```python
from build123d import *

# Parameters (mm, degrees)
F0_R          = 9
F1_DEPTH      = 25
F2_R          = 5
F3_DEPTH      = 10
F4_R          = 4
F5_DEPTH      = 8
F6_R          = 2
F7_DEPTH      = 9.001
F7_DEPTH_BACK = 9.001
F9_R          = 9.6900130566
F10_DEPTH     = 1
F11_R         = 8.2586159941
F12_DEPTH     = 17.0010001


with BuildPart() as f1:
    # F0 (on Front) → F1 (new body)
    with BuildSketch(Plane.XZ):
        Circle(F0_R)
    extrude(amount=F1_DEPTH)

    # F2 (on face) → F3 (cut)
    with BuildSketch(Plane(origin=(0, 0, 0), x_dir=(-1, 0, 0), z_dir=(0, 1, 0))):
        Circle(F2_R)
    extrude(amount=-F3_DEPTH, mode=Mode.SUBTRACT)

    # F4 (on face) → F5 (cut)
    with BuildSketch(Plane.XZ.offset(25)):
        Circle(F4_R)
    extrude(amount=-F5_DEPTH, mode=Mode.SUBTRACT)

    # F6 (on Right) → F7 (cut, two sides)
    with BuildSketch(Plane.YZ) as f7_sk:
        with Locations((-21, 0)):
            Circle(F6_R)
        with Locations((-4, 0)):
            Circle(F6_R)
    extrude(amount=-F7_DEPTH, mode=Mode.SUBTRACT)
    extrude(f7_sk.sketch, amount=F7_DEPTH_BACK, mode=Mode.SUBTRACT)


with BuildPart() as f10:
    # F9 (on offset) → F10 (new body)
    with BuildSketch(Plane.XZ.offset(8)):
        Circle(F9_R)
    extrude(amount=F10_DEPTH)

    # F11 (on face) → F12 (cut, through all)
    with BuildSketch(Plane(origin=(0, -8, 0), x_dir=(-1, 0, 0), z_dir=(0, 1, 0))):
        Circle(F11_R)
    extrude(amount=-F12_DEPTH, mode=Mode.SUBTRACT)


with BuildPart() as f1_1:
    add(f1.part)

    # F13: cut F10
    add(f10.part, mode=Mode.SUBTRACT)


solid = f1_1.part
```
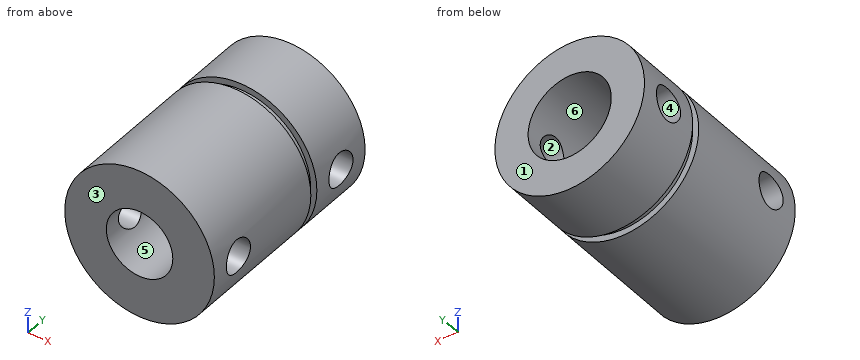
Check sheet for the modelled part. Datum: model origin and axes. Units: mm. Face numbers are marked on the shaded views. A direction names the side the tool comes from. Coordinates: 2 decimals unless noted, no trailing zeros. Write each loop counter-clockwise with the first axis right and the second up, starting at its lowest first coordinate (ties: lowest second). Pieces come first, ordered by that corner, then holes. Notation, with made-up numbers: (34.25, 73) - (74.25, 73) arc R27 cw to (74.25, 106) - close; hole circle Ø5 at (21, -19.75). An arc over 180 degrees is marked (long way). One line per question, with ' | ' between items.
Item 1: Sectioned sample at B-B on x = 7. Record the boundary of the cut face in (y, z).
Determined:
outline: (-25, -5.66) - (-9, -5.66) - (-9, -4.38) - (-8, -4.38) - (-8, -5.66) - (0, -5.66) - (0, 5.66) - (-8, 5.66) - (-8, 4.38) - (-9, 4.38) - (-9, 5.66) - (-25, 5.66) - close; hole circle Ø4 at (-21, 0); hole circle Ø4 at (-4, 0)
Item 2: Gauge pin test, flat ends, axial feed: P1, Ø5, axis at x = 4.5, y = -9.5, coming from the -Z side; P2, Ø1.5, axis at y = -17, z = 3.5, coming from the -X side; P3, Ø7, axis at x = 0, z = 0, coming from the +Y side. Record the tip position at first contact, or that the pin passes through.
Determined:
P1: stops at z = -8.77 | P2: stops at x = -8.57 | P3: stops at y = -10
Item 3: Sectioned sample at D-D on y = -22. Record the boundary of the cut face in (x, z), plus the area to 3 significant figures.
Determined:
outline: (-8.83, -1.73) arc R9 ccw to (8.83, -1.73) - (3.61, -1.73) arc R4 cw to (-3.61, -1.73) - close; (-8.83, 1.73) - (-3.61, 1.73) arc R4 cw to (3.61, 1.73) - (8.83, 1.73) arc R9 ccw to start | area: 169 mm2
Item 4: Access from +Z, -Z, +X, -X, +Y, -Y to the whole of each face (thin tool, end or side, straight path). Record for the marked faces 4, 5 and 6.
Determined:
face 4: +X, -X | face 5: -Y | face 6: +Y
Item 5: Mould release check, pull along Y, two halves, no side actions. Record for the marked faces 1, 2 and 3: pulls with the +Y half, pulls with the -Y half, needs draft (parallel to the pull), parting line crosses it, or undercut.
Determined:
face 1: pulls with the +Y half | face 2: undercut | face 3: pulls with the -Y half
Item 6: Sectioned sample at A-A on y = -4. Record the boundary of the cut face in (x, z).
Determined:
outline: (-8.77, -2) arc R9 ccw to (8.77, -2) - (4.58, -2) arc R5 cw to (-4.58, -2) - close; (-8.77, 2) - (-4.58, 2) arc R5 cw to (4.58, 2) - (8.77, 2) arc R9 ccw to start
Item 7: Sectioned sample at C-C on z = 3. Record the boundary of the cut face in (x, y), plus the area to 3 significant figures.
Determined:
outline: (-8.49, -25) - (-2.65, -25) - (-2.65, -17) - (2.65, -17) - (2.65, -25) - (8.49, -25) - (8.49, -9) - (7.69, -9) - (7.69, -8) - (8.49, -8) - (8.49, 0) - (4, 0) - (4, -10) - (-4, -10) - (-4, 0) - (-8.49, 0) - (-8.49, -8) - (-7.69, -8) - (-7.69, -9) - (-8.49, -9) - close | area: 300 mm2
Item 8: Thickness scan on line 1 (Y direction, x = 6.6, z = 0); line 2 (Y direction, x = 8, z = -2.25); line 3 (Y direction, x = 5, z = 1.25). Record the ranges inside material, lowest first. Write a range as [from, to].
Determined:
line 1: y = [-25, -23], [-19, -6], [-2, 0] | line 2: y = [-25, -9], [-8, 0] | line 3: y = [-25, -22.56], [-19.44, -5.56], [-2.44, 0]
